Can you work these out from the drawing? Everything is in mm from the part's minimum corner. A direction names the side the tool comes from. Round coordinates to 2 decimals unless told otherwise and drop trailing zeros. Write each loop counter-clockwise with the first axis right and the second up, starting at its lowest first coordinate (ties: lowest second). Pieces come first, ordered by that corner, then holes.
Q1. I'm going to push flat-ended pins straight in: pin 1 Ø8 at (x, y) = (17, 5) entering from +Z; pin 2 Ø4 at (x, y) = (8.5, 7) entering from +Z; pin 3 Ø1.5 at (x, y) = (20, 20) entering from +Z (1 decimal); pin 4 Ø8 at (x, z) = (32.5, 32.5) entering from -Y. Where does each tip first touch, or does it pass through?
Q2. If we section it at D-D (z = 44): Please give me the cut outline in (x, y), plus the area to 3 significant figures.
Q3. If we section it at B-B (y = 10.5): Please give me the cut outline in (x, z), plus the area to 3 significant figures.
Q4. If we section it at A-A (z = 32.5): Please give me the cut outline in (x, y), plus the area to 3 significant figures.
Q5. We'd pull the mould along X, two halves only. Please class the marked faces 4, 5 and 6: +X half, -X half, draft (parallel to the pull), parting line (faces both ways), or undercut.
Q6. For the marked faces 1, 2 and 3, which set-ups out of +Z, -Z, +X, -X, +Y, -Y let a thin tool reach every point of the face, with its end or its side?
Q7. Please list where these lines run through material, in increasing order: line 1 along Y through (x, z) = (8.5, 38); line 2 along Z through (x, y) = (36.5, 20.75) (1 decimal); line 3 along Z through (x, y) = (21, 9.25).
Q8. If we section it at C-C (x = 32.5): Please give me the cut outline in (y, z).
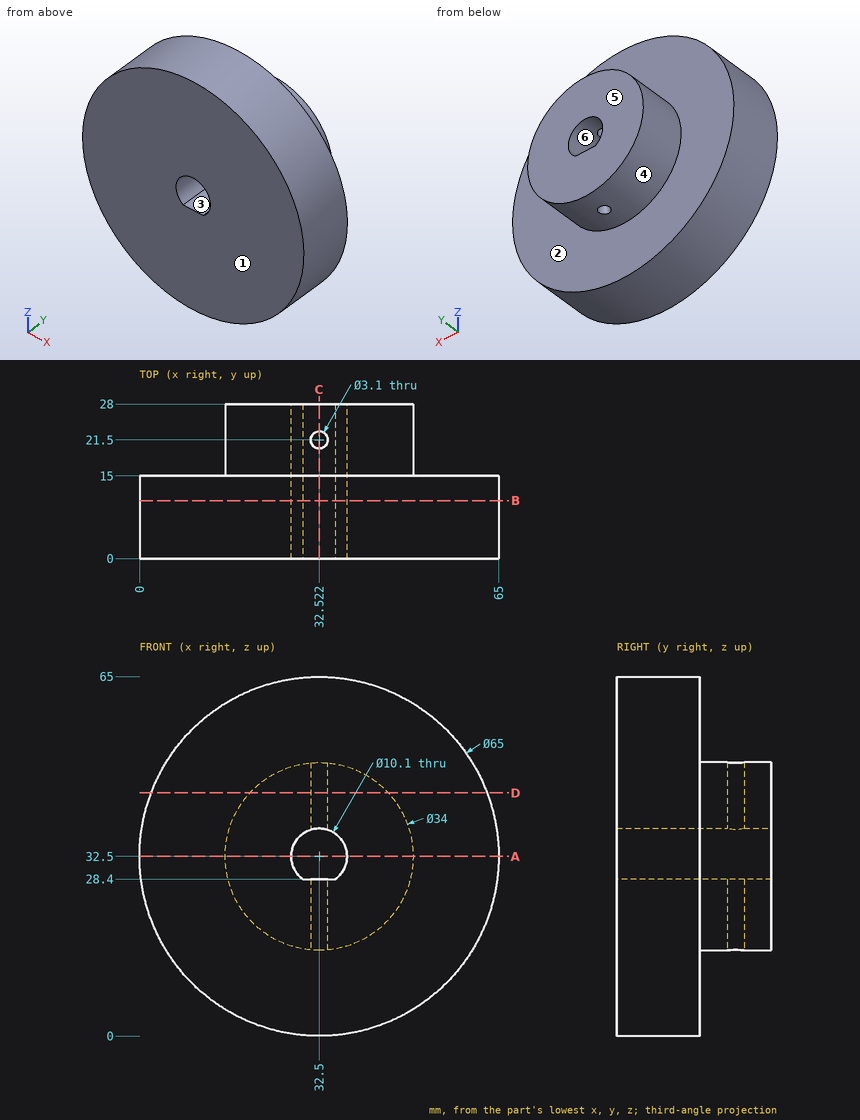
A:
1. pin 1: stops at z = 62.9
1. pin 2: stops at z = 56.42
1. pin 3: stops at z = 44.8
1. pin 4: passes through
2. outline: (2.1, 0) - (62.9, 0) - (62.9, 15) - (45.02, 15) - (45.02, 28) - (19.98, 28) - (19.98, 15) - (2.1, 15) - close; hole circle Ø3.1 at (32.52, 21.5)
2. area: 1,230 mm2
3. outline: circle Ø65 at (32.5, 32.5); hole (29.55, 28.4) - (35.45, 28.4) arc R5.05 ccw (long way) to start
3. area: 3,240 mm2
4. outline: (0, 0) - (27.45, 0) - (27.45, 28) - (15.5, 28) - (15.5, 15) - (0, 15) - close; (37.55, 0) - (65, 0) - (65, 15) - (49.5, 15) - (49.5, 28) - (37.55, 28) - close
4. area: 1,130 mm2
5. face 4: parting line
5. face 5: draft
5. face 6: undercut
6. face 1: +Z, -Z, +X, -X, -Y
6. face 2: +Y
6. face 3: +Y, -Y
7. line 1: y = 0 to 15
7. line 2: z = 16 to 29.4, 35.6 to 49
7. line 3: z = 2.1 to 62.9
8. outline: (0, 0) - (15, 0) - (15, 15.5) - (19.95, 15.5) - (19.95, 28.4) - (0, 28.4) - close; (0, 37.55) - (19.95, 37.55) - (19.95, 49.5) - (15, 49.5) - (15, 65) - (0, 65) - close; (23.05, 15.5) - (28, 15.5) - (28, 28.4) - (23.05, 28.4) - close; (23.05, 37.55) - (28, 37.55) - (28, 49.5) - (23.05, 49.5) - close
